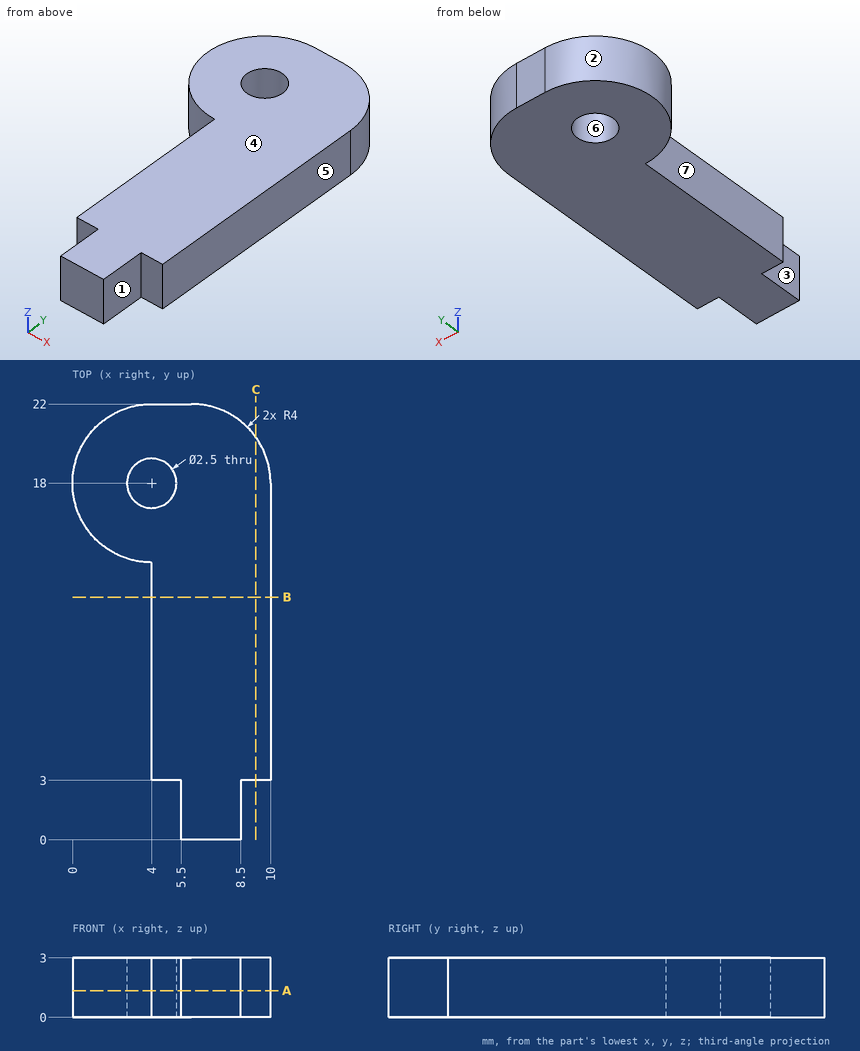
Can you work these out from the drawing? Everything is in mm from the part's minimum corner. A direction names the side the tool comes from. Give positions to 0.01 mm unless a question says otherwise; leave off trailing zeros. Loops run counter-clockwise (first coordinate to the right, second up) from the corner with the lowest first, then second, coordinate; pieces in that order, holes last. Notation, with made-up numbers: (2.5, 86) -> (10.5, 86) arc R23 cw to (10.5, 119) -> close; hole circle Ø1 at (-32.75, 77.5). An arc over 180 degrees is marked (long way). Return JSON: item names as keys, results as strings.
Q1. I want a section at A-A, the plane z = 1.35. List the corners of the cut face in (x, y) for me.
Checks:
{"outline": "(4, 3) -> (5.5, 3) -> (5.5, 0) -> (8.5, 0) -> (8.5, 3) -> (10, 3) -> (10, 18) arc R4 ccw to (6, 22) -> (4, 22) arc R4 ccw to (4, 14) -> close; hole circle Ø2.5 at (4, 18)"}
Q2. For pin 1 Ø1.5 at (y, z) = (2, 1.5) entering from +X; pin 2 Ø1.6 at (x, z) = (9.5, 2) entering from -Y; pin 3 Ø1.5 at (y, z) = (7.5, 1.5) entering from -X; pin 4 Ø2 at (x, y) = (6.5, 6.5) entering from -Z, each with a flat end and sliding along its axis, tell me the tip position at first contact or that it passes through.
Checks:
{"pin 1": "stops at x = 8.5", "pin 2": "stops at y = 3", "pin 3": "stops at x = 4", "pin 4": "stops at z = 0"}
Q3. We'd pull the mould along X, two halves only. Please class the marked faces 4, 5, 6 and 7: released by +X, released by -X, zero draft, split by the parting line, or undercut.
Checks:
{"face 4": "zero draft", "face 5": "released by +X", "face 6": "undercut", "face 7": "released by -X"}
Q4. I need wall thicknesses on probe 1 along X at (y, z) = (8.5, 1.75); probe 2 along Y at (x, z) = (0.75, 1.15); probe 3 along X at (y, z) = (16.5, 2.4). Which ranges of each line are inside material? Lowest first, please.
Checks:
{"probe 1": "x = 4 to 10", "probe 2": "y = 15.67 to 20.33", "probe 3": "x = 0.29 to 10"}
Q5. I want a section at B-B, the plane y = 12.25. List the corners of the cut face in (x, z) for me, then the cut area to 3 significant figures.
Checks:
{"outline": "(4, 0) -> (10, 0) -> (10, 3) -> (4, 3) -> close", "area": "18.0 mm2"}
Q6. On a 3-axis mill with a long thin cutter (end or side, diameter ignored), from which of +Z, -Z, +X, -X, +Y, -Y can I reach the whole of each face in a straight line? I mean the marked faces 1, 2 and 3. Say none if no direction works.
Checks:
{"face 1": "+Z, -Z, +X, -Y", "face 2": "+Z, -Z, -X", "face 3": "+Z, -Z, -X, -Y"}
Q7. I want a section at C-C, the plane x = 9.25. List the corners of the cut face in (y, z) for me.
Checks:
{"outline": "(3, 0) -> (20.33, 0) -> (20.33, 3) -> (3, 3) -> close"}
